Part model, mm, in its own coordinate system. A direction names the side the tool comes from. Give positions to 0.01 mm unless a question says otherwise; leave off trailing zeros. Order: outer loops, then holes, each group sorted by start corner. A loop starts at its lowest first (then second) coordinate and runs counter-clockwise, first axis right, second up. Notation, with made-up numbers: (14.5, 61) - (22.5, 61) arc R18 cw to (22.5, 89) - close; hole circle Ø2 at (-7, 54.5). An arc over 180 degrees is marked (long way). One line per item, written item: value.
```python
from build123d import *

# Parameters (mm, degrees)
HEX_PART_DEPTH   = 8
SKETCH2_R        = 1.5
THREAD_DEPTH     = 6
SKETCH3_R        = 1.5
HEX_THREAD_DEPTH = 6


with BuildPart() as part:
    # Sketch1 → HEX PART (new body)
    with BuildSketch(Plane(origin=(0, 0, 0), x_dir=(1, 0, 0), z_dir=(0, 1, 0))):
        Polygon((2.655811238, 0), (1.327905619, 2.3), (-1.327905619, 2.3), (-2.655811238, 0), (-1.327905619, -2.3), (1.327905619, -2.3), align=None)
    extrude(amount=HEX_PART_DEPTH)

    # Sketch2 → THREAD (add)
    with BuildSketch(Plane(origin=(0, 0, 0), x_dir=(1, 0, 0), z_dir=(0, 1, 0))):
        with Locations(Location((0, 0, 0), (0, 0, 270))):
            Circle(SKETCH2_R)
    extrude(amount=-THREAD_DEPTH)

    # Sketch3 → HEX THREAD (cut)
    with BuildSketch(Plane(origin=(0, 8, 0), x_dir=(1, 0, 0), z_dir=(0, 1, 0))):
        with Locations(Location((0, 0, 0), (0, 0, 270))):
            Circle(SKETCH3_R)
    extrude(amount=-HEX_THREAD_DEPTH, mode=Mode.SUBTRACT)


solid = part.part
```
1) Mould opens along Z. For faces 1 (the flat face through (0, 2, 0)), 2 (the flat face through (-1.98, 3.94, -1.17)), 3 (the flat face through (0, 0, -2)), 4 (the flat face through (0, 4, 2.3)) say: released by +Z, released by -Z, zero draft, split by the parting line, or undercut.
Outcome:
face 1: undercut
face 2: released by -Z
face 3: zero draft
face 4: released by +Z
2) Which spindle directions (+Z, -Z, +X, -X, +Y, -Y) get a long thin tool onto all of the face, cutting with end or side? Do faces 5 (the cylindrical face through (0.45, -2.96, 1.43)), 6 (the flat face through (0, 8, -2)), 7 (the cylindrical face through (0.45, 5.04, 1.43)). Say none if no direction does.
Outcome:
face 5: -Y
face 6: +Z, -Z, +X, -X, +Y
face 7: +Y
3) Cut at A-A, the plane y = 0.5. Give the cut face in (x, z), then the cut area to 3 significant figures.
Outcome:
outline: (-2.66, 0) - (-1.33, -2.3) - (1.33, -2.3) - (2.66, 0) - (1.33, 2.3) - (-1.33, 2.3) - close
area: 18.3 mm^2
4) Cut at C-C, the plane z = 0.6. Give the cut face in (x, y), then the cut area to 3 significant figures.
Outcome:
outline: (-2.31, 0) - (-1.37, 0) - (-1.37, -6) - (1.37, -6) - (1.37, 0) - (2.31, 0) - (2.31, 8) - (1.37, 8) - (1.37, 2) - (-1.37, 2) - (-1.37, 8) - (-2.31, 8) - close
area: 37.0 mm^2
5) Cut at D-D, the plane z = 1.95. Give the cut face in (x, y), then the cut area to 3 significant figures.
Outcome:
outline: (-1.53, 0) - (1.53, 0) - (1.53, 8) - (-1.53, 8) - close
area: 24.5 mm^2
6) Drill centre lines: line 1 along Y through (x, z) = (-1, 1.55); line 2 along Y through (x, z) = (-0.65, -0.3); line 3 along X through (y, z) = (2.25, -2). Where is each one in solid material? Low to high. Write a range as from..to.
Outcome:
line 1: y = 0..8
line 2: y = -6..2
line 3: x = -1.5..1.5
7) Cut at B-B, the plane x = 0. Give the cut face in (y, z), then the cut area to 3 significant figures.
Outcome:
outline: (-6, -1.5) - (0, -1.5) - (0, -2.3) - (8, -2.3) - (8, -1.5) - (2, -1.5) - (2, 1.5) - (8, 1.5) - (8, 2.3) - (0, 2.3) - (0, 1.5) - (-6, 1.5) - close
area: 36.8 mm^2
